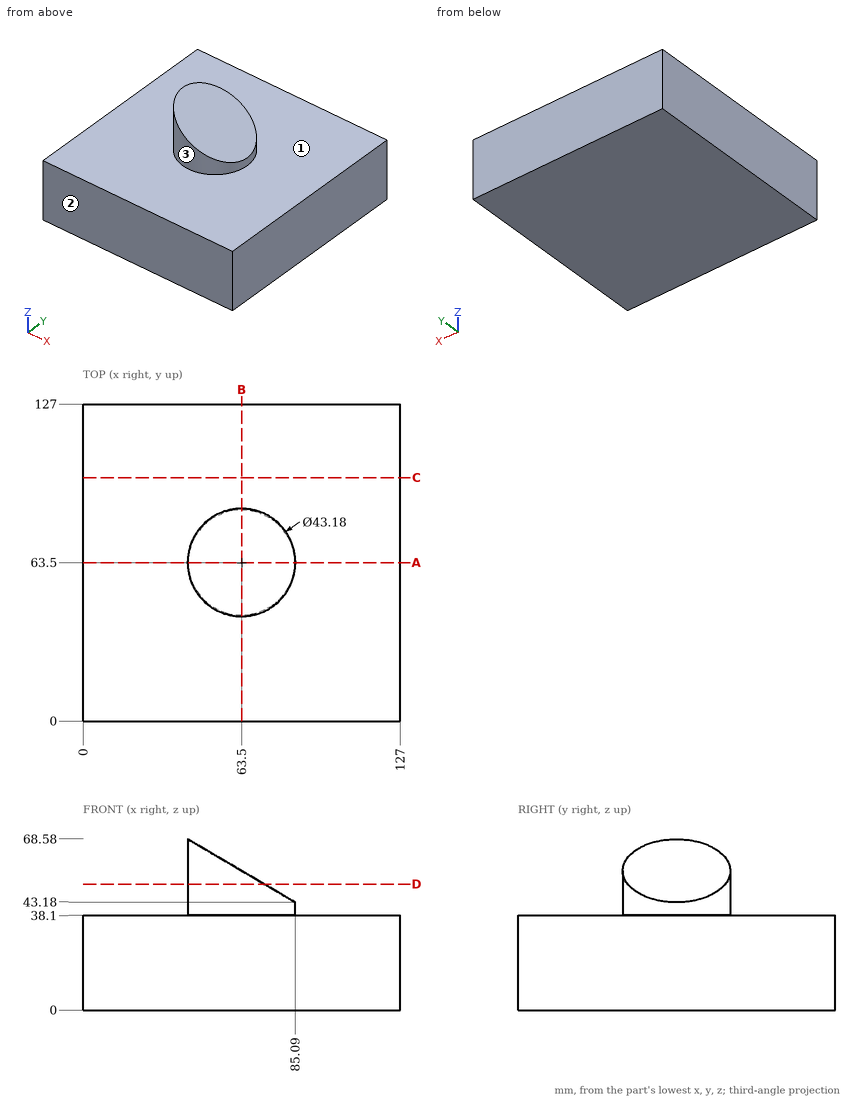
Part print with two shaded views. Sizes in mm from the minimum x, y, z corner. Round coordinates to 2 decimals unless told otherwise and drop trailing zeros. Write each loop counter-clockwise with the first axis right and the second up, starting at its lowest first coordinate (ties: lowest second). Pieces come first, ordered by that corner, then holes. Notation, with made-up numbers: M 18.25,-29.75 L 30.25,-29.75 A26 cw 30.25,-4.75 Z; hole C -24.75,82.25 d8. An arc over 180 degrees is marked long. Put each result on its own line as item: value. Start each with the question number.
1) Saw through at A-A, the plane y = 63.5. Write the cut outline in (x, z), and give its area (3 significant figures).
2) Saw through at B-B, the plane x = 63.5. Write the cut outline in (y, z).
3) Pin check, flat tips, straight feed: pin 1 Ø4 at (x, y) = (14, 107.5) entering from -Z; pin 2 Ø6 at (y, z) = (47.5, 59.5) entering from -X; pin 3 Ø10 at (y, z) = (38.5, 48) entering from -X; pin 4 Ø1 at (x, y) = (113.5, 35.5) entering from +Z. Stop position of each tip, or through.
4) Drill centre lines: probe 1 along Z at (x, y) = (100.5, 117.5); probe 2 along Z at (x, y) = (75.5, 75). Where is each one in solid material? Low to high. Write a range as [from, to].
5) Saw through at D-D, the plane z = 50.5. Write the cut outline in (x, y).
6) Pull direction Y, two halves, no side cores. Call the marked faces 1, 2 and 3: pulls with the +Y half, pulls with the -Y half, needs draft (parallel to the pull), parting line crosses it, or undercut.
7) Saw through at C-C, the plane y = 97.5. Write the cut outline in (x, z).
Resolved:
1. outline: M 0,0 L 127,0 L 127,38.1 L 85.09,38.1 L 85.09,43.18 L 41.91,68.58 L 41.91,38.1 L 0,38.1 Z
1. area: 5,610 mm²
2. outline: M 0,0 L 127,0 L 127,38.1 L 85.09,38.1 L 85.09,55.88 L 41.91,55.88 L 41.91,38.1 L 0,38.1 Z
3. pin 1: z = 0
3. pin 2: x = 46.26
3. pin 3: x = 55.37
3. pin 4: z = 38.1
4. probe 1: [0, 38.1]
4. probe 2: [0, 48.82]
5. outline: M 72.65,43.94 L 72.65,83.06 A21.59 ccw long Z
6. face 1: needs draft
6. face 2: pulls with the -Y half
6. face 3: parting line crosses it
7. outline: M 0,0 L 127,0 L 127,38.1 L 0,38.1 Z
